```python
from build123d import *

# Parameters (mm, degrees)
SKETCH3_R           = 2.54
BOSS_EXTRUDE1_DEPTH = 10
SKETCH2_R           = 2.54
SKETCH2_R_2         = 12.7
BOSS_EXTRUDE2_DEPTH = 6
SKETCH4_R           = 12.7
SKETCH4_R_2         = 2.54
BOSS_EXTRUDE3_DEPTH = 8
SKETCH5_R           = 2.38125
CUT_EXTRUDE1_DEPTH  = 70


with BuildPart() as part:
    # Sketch3 → Boss-Extrude1 (new body)
    with BuildSketch(Plane(origin=(0, 0, 0), x_dir=(0, 0, -1), z_dir=(1, 0, 0))):
        with BuildLine():
            Line((32.460000001, 26), (32.460000001, 17))
            Line((32.460000001, 17), (22.011694736, 17))
            ThreePointArc((22.011694736, 17), (20.785715032, 16.58018156), (20.074424214, 15.496973764))
            Line((20.074424214, 15.496973764), (11.242399458, -18.931445665))
            ThreePointArc((11.242399458, -18.931445665), (0.051229837, -22.017914435), (-11.154181322, -18.983556558))
            Line((-11.154181322, -18.983556558), (-20.149993239, 15.504783566))
            ThreePointArc((-20.149993239, 15.504783566), (-20.862453065, 16.582650803), (-22.085243494, 17))
            Line((-22.085243494, 17), (-32.539999999, 17))
            Line((-32.539999999, 17), (-32.539999999, 26))
            ThreePointArc((-32.539999999, 26), (-31.368427124, 28.828427124), (-28.539999999, 30))
            Line((-28.539999999, 30), (28.460000001, 30))
            ThreePointArc((28.460000001, 30), (31.288427125, 28.828427124), (32.460000001, 26))
        make_face()
        with Locations((-23.5712, 23.5712)):
            Circle(SKETCH3_R, mode=Mode.SUBTRACT)
        with Locations((23.5712, 23.5712)):
            Circle(SKETCH3_R, mode=Mode.SUBTRACT)
        with BuildLine():
            Line((-9.365008666, 1.738431537), (-6.243342957, 18.43092489))
            ThreePointArc((-6.243342957, 18.43092489), (-0.00846666, 23.621964814), (6.240230217, 18.447569655))
            Line((6.240230217, 18.447569655), (9.360339559, 1.763398668))
            ThreePointArc((9.360339559, 1.763398668), (0.012699982, -9.524986626), (-9.365008666, 1.738431537))
        make_face(mode=Mode.SUBTRACT)
    extrude(amount=BOSS_EXTRUDE1_DEPTH)

    # Sketch2 → Boss-Extrude2 (add)
    with BuildSketch(Plane(origin=(10, 0, 0), x_dir=(0, 0, -1), z_dir=(1, 0, 0))):
        with BuildLine():
            Line((-28.5, 30), (28.5, 30))
            ThreePointArc((28.5, 30), (31.328427125, 28.828427125), (32.5, 26))
            Line((32.5, 26), (32.5, -26))
            ThreePointArc((32.5, -26), (31.328427125, -28.828427125), (28.5, -30))
            Line((28.5, -30), (-28.5, -30))
            ThreePointArc((-28.5, -30), (-31.328427125, -28.828427125), (-32.5, -26))
            Line((-32.5, -26), (-32.5, 26))
            ThreePointArc((-32.5, 26), (-31.328427125, 28.828427125), (-28.5, 30))
        make_face()
        with Locations((-23.5712, 23.5712)):
            Circle(SKETCH2_R, mode=Mode.SUBTRACT)
        with Locations((23.5712, 23.5712)):
            Circle(SKETCH2_R, mode=Mode.SUBTRACT)
        with Locations((23.5712, -23.5712)):
            Circle(SKETCH2_R, mode=Mode.SUBTRACT)
        with Locations(Location((0, 0, 0), (0, 0, 127.997746865))):
            Circle(SKETCH2_R_2, mode=Mode.SUBTRACT)
        with Locations((-23.5712, -23.5712)):
            Circle(SKETCH2_R, mode=Mode.SUBTRACT)
        with BuildLine():
            Line((25.1, 2), (25.1, -2))
            ThreePointArc((25.1, -2), (27.48125, -4.38125), (29.8625, -2))
            Line((29.8625, -2), (29.8625, 2))
            ThreePointArc((29.8625, 2), (27.48125, 4.38125), (25.1, 2))
        make_face(mode=Mode.SUBTRACT)
        with BuildLine():
            Line((-29.8625, -2), (-29.8625, 2))
            ThreePointArc((-29.8625, 2), (-27.48125, 4.38125), (-25.1, 2))
            Line((-25.1, 2), (-25.1, -2))
            ThreePointArc((-25.1, -2), (-27.48125, -4.38125), (-29.8625, -2))
        make_face(mode=Mode.SUBTRACT)
    extrude(amount=BOSS_EXTRUDE2_DEPTH)

    # Sketch4 → Boss-Extrude3 (add)
    with BuildSketch(Plane(origin=(16, 0, 0), x_dir=(0, 0, -1), z_dir=(1, 0, 0))):
        with BuildLine():
            Line((-28.448, -7.771660717), (-28.448, -23.6855))
            ThreePointArc((-28.448, -23.6855), (-27.053096045, -27.053096045), (-23.6855, -28.448))
            Line((-23.6855, -28.448), (23.6855, -28.448))
            ThreePointArc((23.6855, -28.448), (27.053096045, -27.053096045), (28.448, -23.6855))
            Line((28.448, -23.6855), (28.448, -7.771660717))
            ThreePointArc((28.448, -7.771660717), (28.699853039, -6.800073252), (29.391982202, -6.073183043))
            ThreePointArc((29.391982202, -6.073183043), (30.644303408, -4.75796607), (31.1, -3))
            Line((31.1, -3), (31.1, 3))
            ThreePointArc((31.1, 3), (30.644303408, 4.75796607), (29.391982202, 6.073183043))
            ThreePointArc((29.391982202, 6.073183043), (28.699853039, 6.800073252), (28.448, 7.771660717))
            Line((28.448, 7.771660717), (28.448, 23.6855))
            ThreePointArc((28.448, 23.6855), (27.053096045, 27.053096045), (23.6855, 28.448))
            Line((23.6855, 28.448), (-23.6855, 28.448))
            ThreePointArc((-23.6855, 28.448), (-27.053096045, 27.053096045), (-28.448, 23.6855))
            Line((-28.448, 23.6855), (-28.448, 7.771660717))
            ThreePointArc((-28.448, 7.771660717), (-28.699853039, 6.800073252), (-29.391982202, 6.073183043))
            ThreePointArc((-29.391982202, 6.073183043), (-30.644303408, 4.75796607), (-31.1, 3))
            Line((-31.1, 3), (-31.1, -3))
            ThreePointArc((-31.1, -3), (-30.644303408, -4.75796607), (-29.391982202, -6.073183043))
            ThreePointArc((-29.391982202, -6.073183043), (-28.699853039, -6.800073252), (-28.448, -7.771660717))
        make_face()
        with Locations(Location((0, 0, 0), (0, 0, 127.997746865))):
            Circle(SKETCH4_R, mode=Mode.SUBTRACT)
        with Locations((23.5712, 23.5712)):
            Circle(SKETCH4_R_2, mode=Mode.SUBTRACT)
        with Locations((-23.5712, 23.5712)):
            Circle(SKETCH4_R_2, mode=Mode.SUBTRACT)
        with Locations((23.5712, -23.5712)):
            Circle(SKETCH4_R_2, mode=Mode.SUBTRACT)
        with Locations((-23.5712, -23.5712)):
            Circle(SKETCH4_R_2, mode=Mode.SUBTRACT)
        with BuildLine():
            Line((-15.624180672, 23.6855), (-5.175, 23.6855))
            ThreePointArc((-5.175, 23.6855), (-3.760786438, 23.099713562), (-3.175, 21.6855))
            Line((-3.175, 21.6855), (-3.175, 18.200129406))
            ThreePointArc((-3.175, 18.200129406), (-3.39755641, 17.283235582), (-4.015694283, 16.570402356))
            Line((-4.015694283, 16.570402356), (-8.206292299, 13.589422052))
            ThreePointArc((-8.206292299, 13.589422052), (-9.481700161, 13.316114711), (-10.654369458, 13.887261661))
            Line((-10.654369458, 13.887261661), (-17.038394234, 20.271286438))
            ThreePointArc((-17.038394234, 20.271286438), (-17.471939737, 22.450866865), (-15.624180672, 23.6855))
        make_face(mode=Mode.SUBTRACT)
        with BuildLine():
            Line((23.6855, 15.624180672), (23.6855, -15.624180672))
            ThreePointArc((23.6855, -15.624180672), (22.450866865, -17.471939737), (20.271286438, -17.038394234))
            Line((20.271286438, -17.038394234), (13.887261661, -10.654369458))
            ThreePointArc((13.887261661, -10.654369458), (13.316114711, -9.481700161), (13.589422052, -8.206292299))
            ThreePointArc((13.589422052, -8.206292299), (15.875, 0), (13.589422052, 8.206292299))
            ThreePointArc((13.589422052, 8.206292299), (13.316114711, 9.481700161), (13.887261661, 10.654369458))
            Line((13.887261661, 10.654369458), (20.271286438, 17.038394234))
            ThreePointArc((20.271286438, 17.038394234), (22.450866865, 17.471939737), (23.6855, 15.624180672))
        make_face(mode=Mode.SUBTRACT)
        with BuildLine():
            Line((17.038394234, -20.271286438), (10.654369458, -13.887261661))
            ThreePointArc((10.654369458, -13.887261661), (9.481700161, -13.316114711), (8.206292299, -13.589422052))
            Line((8.206292299, -13.589422052), (4.015694283, -16.570402356))
            ThreePointArc((4.015694283, -16.570402356), (3.39755641, -17.283235582), (3.175, -18.200129406))
            Line((3.175, -18.200129406), (3.175, -21.6855))
            ThreePointArc((3.175, -21.6855), (3.760786438, -23.099713562), (5.175, -23.6855))
            Line((5.175, -23.6855), (15.624180672, -23.6855))
            ThreePointArc((15.624180672, -23.6855), (17.471939737, -22.450866865), (17.038394234, -20.271286438))
        make_face(mode=Mode.SUBTRACT)
        with BuildLine():
            Line((-23.6855, -15.624180672), (-23.6855, 15.624180672))
            ThreePointArc((-23.6855, 15.624180672), (-22.450866865, 17.471939737), (-20.271286438, 17.038394234))
            Line((-20.271286438, 17.038394234), (-13.887261661, 10.654369458))
            ThreePointArc((-13.887261661, 10.654369458), (-13.316114711, 9.481700161), (-13.589422052, 8.206292299))
            ThreePointArc((-13.589422052, 8.206292299), (-15.875, 0), (-13.589422052, -8.206292299))
            ThreePointArc((-13.589422052, -8.206292299), (-13.316114711, -9.481700161), (-13.887261661, -10.654369458))
            Line((-13.887261661, -10.654369458), (-20.271286438, -17.038394234))
            ThreePointArc((-20.271286438, -17.038394234), (-22.450866865, -17.471939737), (-23.6855, -15.624180672))
        make_face(mode=Mode.SUBTRACT)
        with BuildLine():
            Line((17.038394234, 20.271286438), (10.654369458, 13.887261661))
            ThreePointArc((10.654369458, 13.887261661), (9.481700161, 13.316114711), (8.206292299, 13.589422052))
            Line((8.206292299, 13.589422052), (4.015694283, 16.570402356))
            ThreePointArc((4.015694283, 16.570402356), (3.39755641, 17.283235582), (3.175, 18.200129406))
            Line((3.175, 18.200129406), (3.175, 21.6855))
            ThreePointArc((3.175, 21.6855), (3.760786438, 23.099713562), (5.175, 23.6855))
            Line((5.175, 23.6855), (15.624180672, 23.6855))
            ThreePointArc((15.624180672, 23.6855), (17.471939737, 22.450866865), (17.038394234, 20.271286438))
        make_face(mode=Mode.SUBTRACT)
        with BuildLine():
            Line((-3.175, -21.6855), (-3.175, -18.200129406))
            ThreePointArc((-3.175, -18.200129406), (-3.39755641, -17.283235582), (-4.015694283, -16.570402356))
            Line((-4.015694283, -16.570402356), (-8.206292299, -13.589422052))
            ThreePointArc((-8.206292299, -13.589422052), (-9.481700161, -13.316114711), (-10.654369458, -13.887261661))
            Line((-10.654369458, -13.887261661), (-17.038394234, -20.271286438))
            ThreePointArc((-17.038394234, -20.271286438), (-17.471939737, -22.450866865), (-15.624180672, -23.6855))
            Line((-15.624180672, -23.6855), (-5.175, -23.6855))
            ThreePointArc((-5.175, -23.6855), (-3.760786438, -23.099713562), (-3.175, -21.6855))
        make_face(mode=Mode.SUBTRACT)
        with BuildLine():
            Line((25.1, 2), (25.1, -2))
            ThreePointArc((25.1, -2), (27.48125, -4.38125), (29.8625, -2))
            Line((29.8625, -2), (29.8625, 2))
            ThreePointArc((29.8625, 2), (27.48125, 4.38125), (25.1, 2))
        make_face(mode=Mode.SUBTRACT)
        with BuildLine():
            Line((-29.8625, -2), (-29.8625, 2))
            ThreePointArc((-29.8625, 2), (-27.48125, 4.38125), (-25.1, 2))
            Line((-25.1, 2), (-25.1, -2))
            ThreePointArc((-25.1, -2), (-27.48125, -4.38125), (-29.8625, -2))
        make_face(mode=Mode.SUBTRACT)
    extrude(amount=BOSS_EXTRUDE3_DEPTH)

    # Sketch5 → Cut-Extrude1 (cut)
    with BuildSketch(Plane(origin=(0, 30, 0), x_dir=(-1, 0, 0), z_dir=(0, 1, 0))):
        with Locations(Location((-5, -12.7, 0), (0, 0, 90))):
            Circle(SKETCH5_R)
        with Locations(Location((-5, 12.7, 0), (0, 0, 90))):
            Circle(SKETCH5_R)
    extrude(amount=-CUT_EXTRUDE1_DEPTH, mode=Mode.SUBTRACT)


solid = part.part
```
Here's how the part is built. I have some questions about the finished solid (model axes, mm). A direction names the side the tool comes from. Give positions to 0.01 mm unless a question says otherwise; leave off trailing zeros. Loops run counter-clockwise (first coordinate to the right, second up) from the corner with the lowest first, then second, coordinate; pieces in that order, holes last. Notation, with made-up numbers: M 78.5,59.25 L 129.5,59.25 A21 ccw 129.5,85.25 Z; hole C -2.75,64.25 d2. An arc over 180 degrees is marked long. Put each result on its own line as item: value. Start each with the question number.
(1) I need wall thicknesses on line 1 along Z through (x, y) = (15, 23); line 2 along Z through (x, y) = (12.5, 4); line 3 along Y through (x, z) = (14.75, -10). Which ranges of each line are inside material? Lowest first, please. Write a range as [from, to].
(2) Will these pins go through, and if not, where does the flat tip stop? pin 1 Ø5 at (x, y) = (12, 1.5) entering from +Z; pin 2 Ø6 at (x, z) = (5.5, -11) entering from +Y; pin 3 Ø2.5 at (x, z) = (22, -11) entering from +Y; pin 4 Ø5 at (x, z) = (3, -27) entering from -Y.
(3) I want a section at B-B on x = 12.5. Please give me the cut outline in (y, z).
(4) For faces 1 (the flat face through (5, 17, 27)), 2 (the cylindrical face through (19.94, 22.48, -17.46)), 3 (the cylindrical face through (12.958, -28.859, 31.297)), 4 (the cylindrical face through (16.9, 4.38, -27.53)), which set-ups out of +Z, -Z, +X, -X, +Y, -Y let a thin tool reach every point of the face, with its end or its side?
(5) I want a section at A-A on z = 0. Please give me the cut outline in (x, y) (3 decimals).
(6) If we mould it in two halves opening along X, with no side actions, what happens to faces 5 (the flat face through (24, 13, 0)), 6 (the cylindrical face through (5.1, 11.12, 10.32)), 7 (the cylindrical face through (19.94, 4.78, 30.63))? For each: +X half, -X half, draft (parallel to the pull), parting line (faces both ways), or undercut.
(7) I want a section at C-C on y = 19.5. State how many separate pieces and enclosed holes the cut face has, then the cut area to 3 significant figures.
Answer block:
1. line 1: [-32.5, -26.05], [-21.1, 21.1], [26.05, 32.5]
1. line 2: [-32.5, -28.77], [-26.19, -12.05], [12.05, 26.19], [28.77, 32.5]
1. line 3: [-30, -7.83], [7.83, 30]
2. pin 1: z = 32.5
2. pin 2: y = 30
2. pin 3: y = 28.45
2. pin 4: y = 17
3. outline: M -30,-28.5 A4 ccw -26,-32.5 L 26,-32.5 A4 ccw 30,-28.5 L 30,28.5 A4 ccw 26,32.5 L -26,32.5 A4 ccw -30,28.5 Z; hole C -23.57,-23.57 d5.08; hole C -23.57,23.57 d5.08; hole C 0,0 d25.4; hole M -2,-29.86 L 2,-29.86 A2.38 ccw 2,-25.1 L -2,-25.1 A2.38 ccw Z; hole M -2,25.1 L 2,25.1 A2.38 ccw 2,29.86 L -2,29.86 A2.38 ccw Z; hole C 23.57,-23.57 d5.08; hole C 23.57,23.57 d5.08
4. face 1: +Z, -X, -Y
4. face 2: +X
4. face 3: +Z, +X, -X, -Y
4. face 4: +X, -X
5. outline: M 0,-22.018 L 10,-22.018 L 10,-30 L 16,-30 L 16,-28.448 L 24,-28.448 L 24,-12.7 L 10,-12.7 L 10,-9.525 L 0,-9.525 Z; M 0,23.622 L 10,23.622 L 10,12.7 L 24,12.7 L 24,28.448 L 16,28.448 L 16,30 L 0,30 Z
6. face 5: +X half
6. face 6: undercut
6. face 7: draft
7. separate pieces: 1
7. enclosed holes: 2
7. area: 1,130 mm^2
